from build123d import *

# Parameters (mm, degrees)
SKETCH4_R           = 28.575
BOSS_EXTRUDE2_DEPTH = 1
SKETCH5_R           = 15.875
CUT_EXTRUDE5_DEPTH  = 2
SKETCH6_R           = 3.175
CUT_EXTRUDE6_DEPTH  = 2
CIRPATTERN1_COUNT   = 8
CUT_EXTRUDE11_DEPTH = 2


with BuildPart() as part:
    # Sketch4 → Boss-Extrude2 (new body)
    with BuildSketch(Plane.XY):
        Circle(SKETCH4_R)
    extrude(amount=BOSS_EXTRUDE2_DEPTH)

    # Sketch5 → Cut-Extrude5 (cut, through all)
    with BuildSketch(Plane.XY.offset(1)):
        Circle(SKETCH5_R)
    extrude(amount=-CUT_EXTRUDE5_DEPTH, mode=Mode.SUBTRACT)

    # Sketch6 → Cut-Extrude6 (cut, through all)
    with BuildSketch(Plane.XY.offset(1)):
        with Locations((22.225, 0)):
            Circle(SKETCH6_R)
    cut_extrude6 = extrude(amount=-CUT_EXTRUDE6_DEPTH, mode=Mode.SUBTRACT)

    # CirPattern1: Cut-Extrude6 ×8 about axis
    cirpattern1_axis = Axis((0, 0, 0), (0, 0, 1))
    for i in range(1, CIRPATTERN1_COUNT):
        add(cut_extrude6.rotate(cirpattern1_axis, i * 360 / CIRPATTERN1_COUNT), mode=Mode.SUBTRACT)

    # Sketch8 → Cut-Extrude11 (cut, through all)
    with BuildSketch(Plane.XY.offset(1)):
        Polygon((29.433830701, 13.566529963), (10.660598601, 5.790402618), (11.632614519, 3.443748605), (30.405846619, 11.219875951), align=None)
        Polygon((12.351510066, 26.500513186), (10.004856053, 27.472529104), (9.518848094, 26.299202097), (11.865502107, 25.327186179), align=None)
        Polygon((-10.004856053, 27.472529104), (-12.351510066, 26.500513186), (-11.865502107, 25.327186179), (-9.518848094, 26.299202097), align=None)
        Polygon((-26.500513186, 12.351510066), (-27.472529104, 10.004856053), (-26.299202097, 9.518848094), (-25.327186179, 11.865502107), align=None)
        Polygon((-27.472529104, -10.004856053), (-26.500513186, -12.351510066), (-25.327186179, -11.865502107), (-26.299202097, -9.518848094), align=None)
        Polygon((-12.351510066, -26.500513186), (-10.004856053, -27.472529104), (-9.518848094, -26.299202097), (-11.865502107, -25.327186179), align=None)
        Polygon((10.004856053, -27.472529104), (12.351510066, -26.500513186), (11.865502107, -25.327186179), (9.518848094, -26.299202097), align=None)
        Polygon((26.500513186, -12.351510066), (27.472529104, -10.004856053), (26.299202097, -9.518848094), (25.327186179, -11.865502107), align=None)
    extrude(amount=-CUT_EXTRUDE11_DEPTH, mode=Mode.SUBTRACT)


solid = part.part
Can you work these out from the model? Positions are in its coordinate system, mm. A direction names the side the tool comes from. Round coordinates to 2 decimals unless told otherwise and drop trailing zeros. Write each loop counter-clockwise with the first axis right and the second up, starting at its lowest first coordinate (ties: lowest second). Pieces come first, ordered by that corner, then holes. Notation, with made-up numbers: M 3,78.5 L 9,78.5 A26 ccw 9,93.5 Z; hole C 78,-2 d1. An arc over 180 degrees is marked long. Use a Markdown table: item, result.
Item 1: I want a section at A-A (y = 0). List the corners of the cut face in (x, z) for me (3 decimals), and give its area (3 significant figures).
Found:
| item | result |
|---|---|
| outline | M -28.575,0 L -25.4,0 L -25.4,1 L -28.575,1 Z; M -19.05,0 L -15.875,0 L -15.875,1 L -19.05,1 Z; M 15.875,0 L 19.05,0 L 19.05,1 L 15.875,1 Z; M 25.4,0 L 28.575,0 L 28.575,1 L 25.4,1 Z |
| area | 12.7 mm2 |
Item 2: Which directions (+Z, -Z, +X, -X, +Y, -Y) give clear straight access to the entire face, cutting with the end or side of a thin tool? Please do faces 4 (the face through (12, -12, 0)), 5 (the face through (20.1, 9.7, 0.5)).
Found:
| item | result |
|---|---|
| face 4 | -Z, +X, -X, +Y, -Y |
| face 5 | +Z, -Z |
Item 3: For pin 1 Ø5 at (x, y) = (-15.72, -15.72) entering from +Z, with a flat end and sliding along its axis, tell me the tip position at first contact or that it passes through.
Found:
| item | result |
|---|---|
| pin 1 | passes through |
Item 4: I want a section at C-C (x = 6.5). List the corners of the cut face in (y, z) for me, and give its area (3 significant figures).
Found:
| item | result |
|---|---|
| outline | M -27.83,0 L -14.48,0 L -14.48,1 L -27.83,1 Z; M 14.48,0 L 27.83,0 L 27.83,1 L 14.48,1 Z |
| area | 26.7 mm2 |
Item 5: I want a section at D-D (y = 10.5). List the corners of the cut face in (x, z) for me, and give its area (3 significant figures).
Found:
| item | result |
|---|---|
| outline | M -25.89,0 L -11.91,0 L -11.91,1 L -25.89,1 Z; M 11.91,0 L 22.03,0 L 22.03,1 L 11.91,1 Z |
| area | 24.1 mm2 |
Item 6: If I drill on line 1 along Y through (x, z) = (20.5, 0.9); line 2 along Y through (x, z) = (14, 0.95); line 3 along X through (y, z) = (-1, 0.5), over which ranges is the centre line in solid material (lowest first)? Write a range as [from, to].
Found:
| item | result |
|---|---|
| line 1 | y = [-19.91, -2.67], [2.67, 7.12], [9.87, 19.91] |
| line 2 | y = [-24.91, -18.39], [-13.04, -7.48], [7.48, 13.04], [18.39, 24.91] |
| line 3 | x = [-28.56, -25.24], [-19.21, -15.84], [15.84, 19.21], [25.24, 28.56] |
Item 7: We'd pull the mould along X, two halves only. Please class faces 1 (the face through (-0.139, -28.575, 0.493)), 2 (the face through (-14.913, -5.441, 0.507)), 3 (the face through (-28.575, 0.139, 0.493)): released by +X, released by -X, zero draft, split by the parting line, or undercut.
Found:
| item | result |
|---|---|
| face 1 | split by the parting line |
| face 2 | undercut |
| face 3 | released by -X |
